For this review, take the finished solid that the model builds, in its own axes (mm). Face numbers are marked on the shaded views. A direction names the side the tool comes from. Coordinates: 2 decimals unless noted, no trailing zeros. Loops run counter-clockwise (first coordinate to the right, second up) from the corner with the lowest first, then second, coordinate; pieces in that order, holes last.
1. Take a section at C-C, the plane x = 8. State the section outline as (y, z) points, then the cut area to 3 significant figures.
2. To check wall thickness, follow probe 1 along Y at (x, z) = (-5, 7); probe 2 along X at (y, z) = (-18, 16.25); probe 3 along X at (y, z) = (14.5, 17). State the ranges of each line that lie inside material, in increasing order.
3. Machinability: for the marked faces 1, 2 and 3, which of the approach directions +Z, -Z, +X, -X, +Y, -Y give a long, thin tool a straight path to every point of the face, cutting with its end or side? Answer none if there is none.
4. Take a section at D-D, the plane z = 1. State the section outline as (x, y) points.
5. Take a section at B-B, the plane z = 14.5. State the section outline as (x, y) points.
6. Take a section at A-A, the plane y = -17. State the section outline as (x, z) points, then the cut area to 3 significant figures.
7. Clearance check with flat-ended pins moving along their axes: P1, Ø10, axis at x = 0.5, z = 14, coming from the -Y side; P2, Ø10, axis at y = -12.5, z = 15, coming from the +X side; P3, Ø1.5, axis at x = -2, z = 11, coming from the +Y side. State where each tip first meets the part, or that it passes through.
8. Mouldability with a two-part tool opening along X and no side actions: class the marked faces 4, 5, 6 and 7 as pulls with the +X half, pulls with the -X half, needs draft (parallel to the pull), parting line crosses it, or undercut.
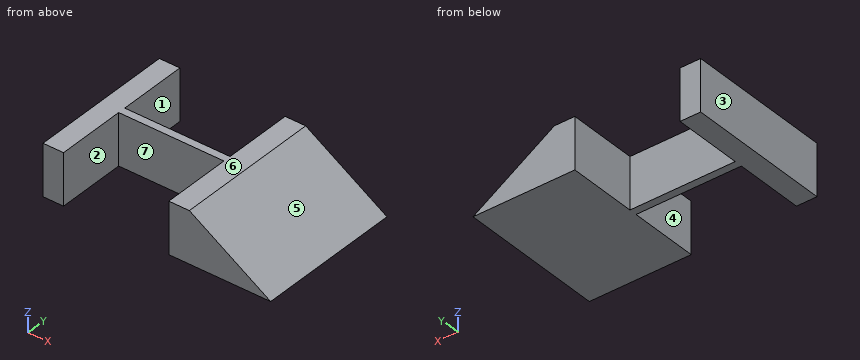
```python
from build123d import *

# Parameters (mm, degrees)
F1_DEPTH = 20
F3_DEPTH = 57


with BuildPart() as f1:
    # F0 (on Top) → F1 (new body)
    with BuildSketch(Plane.XY):
        Polygon((-29.166666, 30), (-37.166666, 30), (-37.166666, -27), (-29.166666, -27), (-29.166666, 0), (11.833334, 0), (11.833334, -27), (19.833334, -27), (19.833334, 30), (11.833334, 30), (11.833334, 3), (-29.166666, 3), align=None)
    extrude(amount=F1_DEPTH)

    # F2 (on face) → F3 (join)
    with BuildSketch(Plane.XZ.offset(27)):
        Polygon((19.833334, 20), (19.833334, 0), (51.504664, 0), align=None)
    extrude(amount=-F3_DEPTH)


solid = f1.part
```
Results list:
1. outline: (0, 0) - (3, 0) - (3, 20) - (0, 20) - close
1. area: 60.0 mm2
2. probe 1: y = 0 to 3
2. probe 2: x = -37.17 to -29.17, 11.83 to 25.77
2. probe 3: x = -37.17 to -29.17, 11.83 to 24.58
3. face 1: +Z, -Z, +Y
3. face 2: +Z, -Z, -Y
3. face 3: +Z, -Z, -X, +Y, -Y
4. outline: (-37.17, -27) - (-29.17, -27) - (-29.17, 0) - (11.83, 0) - (11.83, -27) - (49.92, -27) - (49.92, 30) - (11.83, 30) - (11.83, 3) - (-29.17, 3) - (-29.17, 30) - (-37.17, 30) - close
5. outline: (-37.17, -27) - (-29.17, -27) - (-29.17, 0) - (11.83, 0) - (11.83, -27) - (28.54, -27) - (28.54, 30) - (11.83, 30) - (11.83, 3) - (-29.17, 3) - (-29.17, 30) - (-37.17, 30) - close
6. outline: (-37.17, 0) - (-29.17, 0) - (-29.17, 20) - (-37.17, 20) - close; (11.83, 0) - (51.5, 0) - (19.83, 20) - (11.83, 20) - close
6. area: 637 mm2
7. P1: stops at y = 0
7. P2: stops at x = 35.67
7. P3: stops at y = 3
8. face 4: undercut
8. face 5: pulls with the +X half
8. face 6: needs draft
8. face 7: undercut
